from build123d import *

# Parameters (mm, degrees)
SKETCH_1_R          = 1.5
EXTRUDE_1_DEPTH     = 27.5
SKETCH_2_R          = 1.5
SKETCH_2_R_2        = 1.25
CUT_EXTRUDE_1_DEPTH = 0.4
SKETCH_3_R          = 1.5
SKETCH_3_R_2        = 1.25
CUT_EXTRUDE_2_DEPTH = 0.3
CHAMFER_1_SIZE      = 0.1


with BuildPart() as part:
    # 草图1 → 凸台-拉伸1 (new body)
    with BuildSketch(Plane.XY):
        Circle(SKETCH_1_R)
    extrude(amount=EXTRUDE_1_DEPTH)

    # 草图2 → 切除-拉伸1 (cut)
    with BuildSketch(Plane.XY.offset(0.8)):
        Circle(SKETCH_2_R)
        Circle(SKETCH_2_R_2, mode=Mode.SUBTRACT)
    extrude(amount=CUT_EXTRUDE_1_DEPTH, mode=Mode.SUBTRACT)

    # 草图3 → 切除-拉伸2 (cut)
    with BuildSketch(Plane.XY.offset(26.7)):
        Circle(SKETCH_3_R)
        Circle(SKETCH_3_R_2, mode=Mode.SUBTRACT)
    extrude(amount=-CUT_EXTRUDE_2_DEPTH, mode=Mode.SUBTRACT)

    # 倒角1
    chamfer_1_edges = [part.edges().sort_by_distance(p)[0] for p in [
        (-1.5, 0, 0),
        (-1.5, 0, 27.5),
    ]]
    chamfer(chamfer_1_edges, length=CHAMFER_1_SIZE)


solid = part.part
Can you work these out from the model? Positions are in its coordinate system, mm. A direction names the side the tool comes from. Coordinates: 2 decimals unless noted, no trailing zeros. Write each loop counter-clockwise with the first axis right and the second up, starting at its lowest first coordinate (ties: lowest second). Pieces come first, ordered by that corner, then holes.
Q1. For P1, Ø1, axis at x = 1, z = 6.5, coming from the -Y side; P2, Ø1.5, axis at y = -1, z = 20.5, coming from the -X side; P3, Ø1.5, axis at x = 1, z = 23.5, coming from the +Y side, each with a flat end and sliding along its axis, tell me the tip position at first contact or that it passes through.
Results found:
P1: stops at y = -1.41
P2: stops at x = -1.48
P3: stops at y = 1.48
Q2. Imagine slicing it at A-A, the plane z = 6.25. List the corners of the cut face in (x, y) for me.
Results found:
outline: circle Ø3 at (0, 0)
Q3. If we mould it in two halves opening along Z, with no side actions, what happens to faces 1 (the face through (0, 0, 0)), 2 (the face through (-1.5, 0.07, 13.62)), 3 (the face through (-0.27, -1.22, 1))? For each: +Z half, -Z half, draft (parallel to the pull), parting line (faces both ways), or undercut.
Results found:
face 1: -Z half
face 2: draft
face 3: undercut
Q4. Which directions (+Z, -Z, +X, -X, +Y, -Y) give clear straight access to the entire face, cutting with the end or side of a thin tool? Please do faces 4 (the face through (-1.5, 0.07, 27.05)), 5 (the face through (-0.27, -1.22, 26.55)).
Results found:
face 4: +Z, -Z
face 5: none
Q5. Please list where these lines run through material, in increasing order: L1, parallel to Z at x = 0.75, y = 1.05; L2, parallel to Z at x = 0.1, y = 1.45; L3, parallel to Y at x = 0.55, z = 21.
Results found:
L1: z = 0 to 0.8, 1.2 to 26.4, 26.7 to 27.5
L2: z = 0.05 to 0.8, 1.2 to 26.4, 26.7 to 27.45
L3: y = -1.4 to 1.4
